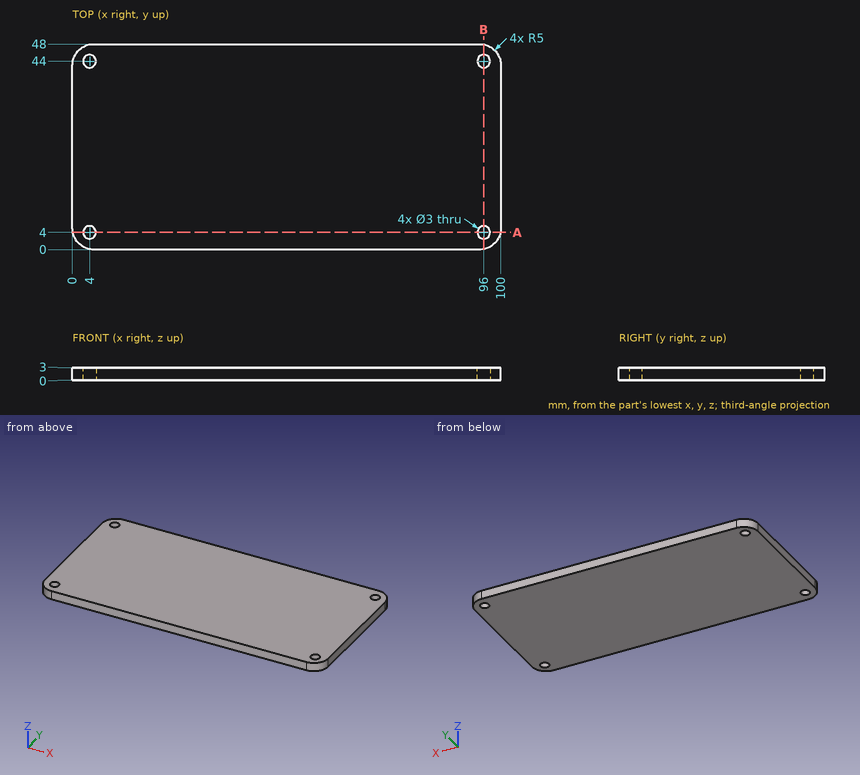
The drawing under review shows one solid part. Ordinate dimensions are in mm from its lowest x, y, z. Coordinates: 2 decimals unless noted, no trailing zeros. Loops run counter-clockwise (first coordinate to the right, second up) from the corner with the lowest first, then second, coordinate; pieces in that order, holes last. Notation, with made-up numbers: (-29.75, 25.25) - (-0.75, 25.25) arc R28 ccw to (-0.75, 60.25) - close; hole circle Ø7 at (-33.75, 50). An arc over 180 degrees is marked (long way). Return JSON: item names as keys, results as strings.
Item 1: For line 1 (Y direction, x = 96, z = 1.3), list the stretches that pass through material, from the lowest coordinate up.
Determined:
{"line 1": "y = 0.1 to 2.5, 5.5 to 42.5, 45.5 to 47.9"}
Item 2: Take a section at A-A (y = 4). Give the boundary of the cut face in (x, z).
Determined:
{"outline": "(0.1, 0) - (2.5, 0) - (2.5, 3) - (0.1, 3) - close; (5.5, 0) - (94.5, 0) - (94.5, 3) - (5.5, 3) - close; (97.5, 0) - (99.9, 0) - (99.9, 3) - (97.5, 3) - close"}
Item 3: Insertion check: pin 1 (3 mm diameter, centred on x = 71.5, y = 22.5, fed in from -Z). The pin has a flat end and moves straight along its axis. Give the tip position at first contact, or say it passes through.
Determined:
{"pin 1": "stops at z = 0"}
Item 4: Take a section at B-B (x = 96). Give the boundary of the cut face in (y, z), then the cut area to 3 significant figures.
Determined:
{"outline": "(0.1, 0) - (2.5, 0) - (2.5, 3) - (0.1, 3) - close; (5.5, 0) - (42.5, 0) - (42.5, 3) - (5.5, 3) - close; (45.5, 0) - (47.9, 0) - (47.9, 3) - (45.5, 3) - close", "area": "125 mm2"}
